```python
from build123d import *

# Parameters (mm, degrees)
F1_DEPTH = 12.7
F2_R     = 0.508


with BuildPart() as f1:
    # F0 (on Front) → F1 (new body)
    with BuildSketch(Plane.XZ):
        with BuildLine():
            Line((-24.592176, 50.020517), (-33.691168, 50.020517))
            Line((-33.691168, 50.020517), (-33.691168, -38.879483))
            Line((-33.691168, -38.879483), (-33.691168, -45.229483))
            Line((-33.691168, -45.229483), (-23.321956, -45.229483))
            Line((-23.321956, -45.229483), (-13.285488, -45.229483))
            ThreePointArc((-13.285488, -45.229483), (-12.903592, -45.170703), (-12.557046, -44.999806))
            Line((-12.557046, -44.999806), (1.165009, -35.391519))
            ThreePointArc((1.165009, -35.391519), (1.680854, -34.605461), (1.514742, -33.680048))
            Line((1.514742, -33.680048), (-0.50165, -30.440789))
            ThreePointArc((-0.50165, -30.440789), (-1.325559, -29.867651), (-2.308267, -30.071614))
            Line((-2.308267, -30.071614), (-14.559193, -38.649806))
            ThreePointArc((-14.559193, -38.649806), (-14.905739, -38.820703), (-15.287635, -38.879483))
            Line((-15.287635, -38.879483), (-22.052176, -38.879483))
            ThreePointArc((-22.052176, -38.879483), (-22.950201, -38.507508), (-23.322176, -37.609483))
            Line((-23.322176, -37.609483), (-23.322176, 29.712342))
            ThreePointArc((-23.322176, 29.712342), (-22.950201, 30.610368), (-22.052176, 30.982342))
            Line((-22.052176, 30.982342), (0.436567, 30.982342))
            ThreePointArc((0.436567, 30.982342), (0.818464, 31.041122), (1.165009, 31.212019))
            Line((1.165009, 31.212019), (10.530465, 37.769782))
            ThreePointArc((10.530465, 37.769782), (11.052137, 38.586245), (10.846207, 39.533001))
            Line((10.846207, 39.533001), (8.677486, 42.665598))
            ThreePointArc((8.677486, 42.665598), (7.857162, 43.192816), (6.90486, 42.983024))
            Line((6.90486, 42.983024), (-0.837138, 37.562019))
            ThreePointArc((-0.837138, 37.562019), (-1.183684, 37.391122), (-1.56558, 37.332342))
            Line((-1.56558, 37.332342), (-22.052176, 37.332342))
            ThreePointArc((-22.052176, 37.332342), (-22.950201, 37.704317), (-23.322176, 38.602342))
            Line((-23.322176, 38.602342), (-23.322176, 48.750517))
            ThreePointArc((-23.322176, 48.750517), (-23.69415, 49.648543), (-24.592176, 50.020517))
        make_face()
    extrude(amount=F1_DEPTH)

    # F2
    f2_edges = [f1.edges().sort_by_distance(p)[0] for p in [
        (-1.183684, -12.7, 37.391122),
        (-11.808878, -12.7, 37.332342),
        (-22.950201, -12.7, 37.704317),
        (-23.322176, -12.7, 43.67643),
        (-23.69415, -12.7, 49.648543),
        (-29.141672, -12.7, 50.020517),
        (-33.691168, -12.7, 2.395517),
        (-23.488328, -12.7, -45.229483),
        (-12.903592, -12.7, -45.170703),
        (-5.696018, -12.7, -40.195662),
        (1.680854, -12.7, -34.605461),
        (0.506546, -12.7, -32.060419),
        (-1.325559, -12.7, -29.867651),
        (-8.43373, -12.7, -34.36071),
        (-14.905739, -12.7, -38.820703),
        (-18.669906, -12.7, -38.879483),
        (-22.950201, -12.7, -38.507508),
        (-23.322176, -12.7, -3.94857),
        (-22.950201, -12.7, 30.610368),
        (-10.807804, -12.7, 30.982342),
        (0.818464, -12.7, 31.041122),
        (5.847737, -12.7, 34.4909),
        (11.052137, -12.7, 38.586245),
        (9.761846, -12.7, 41.0993),
        (7.857162, -12.7, 43.192816),
        (3.033861, -12.7, 40.272522),
        (-1.183684, 0, 37.391122),
        (-11.808878, 0, 37.332342),
        (-22.950201, 0, 37.704317),
        (-23.322176, 0, 43.67643),
        (-23.69415, 0, 49.648543),
        (-29.141672, 0, 50.020517),
        (-33.691168, 0, 2.395517),
        (-23.488328, 0, -45.229483),
        (-12.903592, 0, -45.170703),
        (-5.696018, 0, -40.195662),
        (1.680854, 0, -34.605461),
        (0.506546, 0, -32.060419),
        (-1.325559, 0, -29.867651),
        (-8.43373, 0, -34.36071),
        (-14.905739, 0, -38.820703),
        (-18.669906, 0, -38.879483),
        (-22.950201, 0, -38.507508),
        (-23.322176, 0, -3.94857),
        (-22.950201, 0, 30.610368),
        (-10.807804, 0, 30.982342),
        (0.818464, 0, 31.041122),
        (5.847737, 0, 34.4909),
        (11.052137, 0, 38.586245),
        (9.761846, 0, 41.0993),
        (7.857162, 0, 43.192816),
        (3.033861, 0, 40.272522),
    ]]
    fillet(f2_edges, radius=F2_R)


solid = f1.part
```
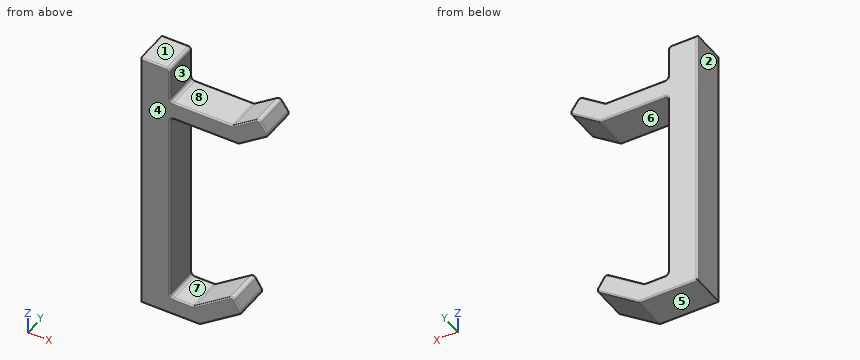
Geometry: final body of the model. Coordinates: model frame, mm. Face numbers are marked on the shaded views. A direction names the side the tool comes from. Round coordinates to 2 decimals unless told otherwise and drop trailing zeros. Loops run counter-clockwise (first coordinate to the right, second up) from the corner with the lowest first, then second, coordinate; pieces in that order, holes last. Notation, with made-up numbers: (8.5, 77.25) -> (57.5, 77.25) arc R31 cw to (57.5, 114.25) -> close; hole circle Ø6 at (34.25, 55.25). An arc over 180 degrees is marked (long way). Write each question's results on one line, items separated by ' | '.
Item 1: Pin query (flat end, axial travel): pin 1 Ø3 at (y, z) = (-5, 42) entering from +X; pin 2 Ø3.5 at (x, y) = (-7.5, -7) entering from +Z; pin 3 Ø6 at (x, y) = (-19.5, -2) entering from +Z. Return the tip coordinate at first contact, or that it passes through.
Answers below:
pin 1: stops at x = 10.18 | pin 2: stops at z = 37.33 | pin 3: stops at z = 37.41
Item 2: Set-up query: the marked faces 4, 5, 6, 7 and 8. Return all of +Z, -Z, +X, -X, +Y, -Y with unobstructed straight access to the full face (end or side cutting, diameter ignored); none if empty.
Answers below:
face 4: +Z, -Z, +X, -X, -Y | face 5: -Z, +X, -X, +Y, -Y | face 6: +X, +Y, -Y | face 7: +Y, -Y | face 8: +Z, +Y, -Y
Item 3: Cut plane A-A on x = -20.5. Return the cut outline in (y, z).
Answers below:
outline: (-12.7, -44.72) arc R0.51 ccw to (-12.19, -45.23) -> (-0.51, -45.23) arc R0.51 ccw to (0, -44.72) -> (0, -39.39) arc R0.51 ccw to (-0.51, -38.88) -> (-12.19, -38.88) arc R0.51 ccw to (-12.7, -39.39) -> close; (-12.7, 31.49) arc R0.51 ccw to (-12.19, 30.98) -> (-0.51, 30.98) arc R0.51 ccw to (0, 31.49) -> (0, 36.82) arc R0.51 ccw to (-0.51, 37.33) -> (-12.19, 37.33) arc R0.51 ccw to (-12.7, 36.82) -> close
Item 4: Cut plane C-C on y = -5.75. Return the cut outline in (x, z) (1 decimal).
Answers below:
outline: (-33.7, -45.2) -> (-13.3, -45.2) arc R1.3 ccw to (-12.6, -45) -> (1.2, -35.4) arc R1.3 ccw to (1.5, -33.7) -> (-0.5, -30.4) arc R1.3 ccw to (-2.3, -30.1) -> (-14.6, -38.6) arc R1.3 cw to (-15.3, -38.9) -> (-22.1, -38.9) arc R1.3 cw to (-23.3, -37.6) -> (-23.3, 29.7) arc R1.3 cw to (-22.1, 31) -> (0.4, 31) arc R1.3 ccw to (1.2, 31.2) -> (10.5, 37.8) arc R1.3 ccw to (10.8, 39.5) -> (8.7, 42.7) arc R1.3 ccw to (6.9, 43) -> (-0.8, 37.6) arc R1.3 cw to (-1.6, 37.3) -> (-22.1, 37.3) arc R1.3 cw to (-23.3, 38.6) -> (-23.3, 48.8) arc R1.3 ccw to (-24.6, 50) -> (-33.7, 50) -> close
Item 5: Pull-direction query (X, two-part tool) for the marked faces 1, 2 and 3; classes: pulls with the +X half, pulls with the -X half, needs draft (parallel to the pull), parting line crosses it, or undercut.
Answers below:
face 1: needs draft | face 2: pulls with the -X half | face 3: undercut
Item 6: Cut plane B-B on z = -6. Return the cut outline in (x, y), and give its area (3 significant figures).
Answers below:
outline: (-33.69, -12.19) arc R0.51 ccw to (-33.18, -12.7) -> (-23.83, -12.7) arc R0.51 ccw to (-23.32, -12.19) -> (-23.32, -0.51) arc R0.51 ccw to (-23.83, 0) -> (-33.18, 0) arc R0.51 ccw to (-33.69, -0.51) -> close | area: 131 mm²
Item 7: Line query: probe 1 along Z at (x, y) = (-22, -5.25); probe 2 along X at (y, z) = (-11.5, -22.5); probe 3 along Z at (x, y) = (-22.5, -9). Output: solid intervals per line, ascending. Write a range as [from, to].
Answers below:
probe 1: z = [-45.23, -38.88], [30.98, 37.33] | probe 2: x = [-33.69, -23.32] | probe 3: z = [-45.23, -38.8], [30.9, 37.41]
